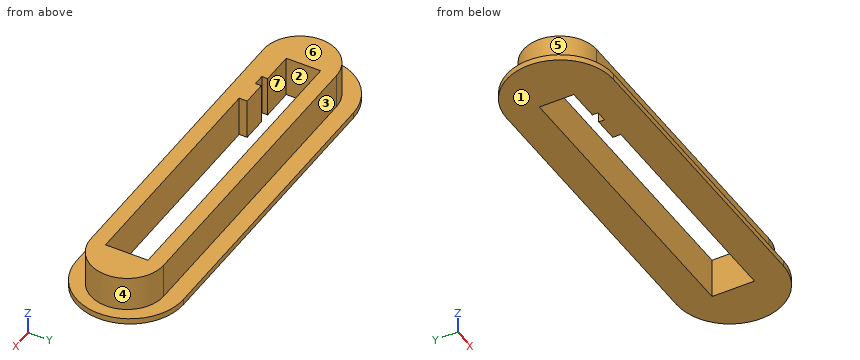
```python
from build123d import *

# Parameters (mm, degrees)
PAD_DEPTH    = 2.1
POCKET_DEPTH = 5
PAD001_DEPTH = 12.5


with BuildPart() as part:
    # Sketch → Pad (new body)
    with BuildSketch(Plane.XY):
        with BuildLine():
            ThreePointArc((0, 19.25), (-19.25, 0), (0, -19.25))
            Line((0, -19.25), (106.5, -19.25))
            ThreePointArc((106.5, -19.25), (125.75, 0), (106.5, 19.25))
            Line((0, 19.25), (106.5, 19.25))
        make_face()
    extrude(amount=PAD_DEPTH)

    # Sketch001 (on Face6 of Pad) → Pocket (cut)
    with BuildSketch(Plane.XY.offset(2.1)):
        Polygon((0.325, 7.65), (108.575, 7.65), (108.575, -7.65), (24.775, -7.65), (24.775, -4.75), (15.975, -4.75), (15.975, -6.85), (11.975, -6.85), (11.975, -4.75), (0.325, -4.75), align=None)
    extrude(amount=-POCKET_DEPTH, mode=Mode.SUBTRACT)

    # Sketch002 (on Face5 of Pocket) → Pad001 (join)
    with BuildSketch(Plane.XY.offset(2.1)):
        with BuildLine():
            ThreePointArc((0, 13.125), (-13.125, 0), (0, -13.125))
            Line((0, -13.125), (108.25, -13.125))
            ThreePointArc((108.25, -13.125), (121.375, 0), (108.25, 13.125))
            Line((0, 13.125), (108.25, 13.125))
        make_face()
        Polygon((0.325, 7.65), (0.325, -4.75), (11.975, -4.75), (11.975, -6.85), (15.975, -6.85), (15.975, -4.75), (24.775, -4.75), (24.775, -7.65), (108.575, -7.65), (108.575, 7.65), align=None, mode=Mode.SUBTRACT)
    extrude(amount=PAD001_DEPTH)


solid = part.part
```
Build history of the part. All positions in model axes, mm. Face numbers are marked on the shaded views. A direction names the side the tool comes from. Round coordinates to 2 decimals unless told otherwise and drop trailing zeros. Loops run counter-clockwise (first coordinate to the right, second up) from the corner with the lowest first, then second, coordinate; pieces in that order, holes last.
Item 1: Two-plate mould, pull along X, no slides. Class the marked faces 4, 5, 6 and 7: released by +X, released by -X, zero draft, split by the parting line, or undercut.
Item 2: Which spindle directions (+Z, -Z, +X, -X, +Y, -Y) get a long thin tool onto all of the face, cutting with end or side? Do the marked faces 1, 2 and 3. Say none if no direction does.
Item 3: Saw through at C-C (z = 7). List the corners of the cut face in (x, y) (3 decimals).
Item 4: Saw through at A-A (y = 0). List the corners of the cut face in (x, z) (3 decimals), then the cut area to 3 significant figures.
Item 5: Saw through at D-D (y = 10). List the corners of the cut face in (x, z), then the cut area to 3 significant figures.
Item 6: Saw through at B-B (x = 104). List the corners of the cut face in (y, z) (3 decimals), then the cut area to 3 significant figures.
Item 7: Pin check, flat tips, straight feed: P1, Ø0.6, axis at y = -6, z = 7, coming from the -X side; P2, Ø8, axis at y = -11.5, z = 1.5, coming from the +X side; P3, Ø6, axis at x = 4.5, z = 9, coming from the +Y side (3 decimals). Stop position of each tip, or through.
Item 8: Drill centre lines: line 1 along Y through (x, z) = (8, 11.25) (3 decimals); line 2 along X through (y, z) = (0.5, 10) (3 decimals); line 3 along Y through (x, z) = (25, 7) (3 decimals). Where is each one in solid material? Low to high.
Worked answers:
1. face 4: released by +X
1. face 5: released by -X
1. face 6: zero draft
1. face 7: undercut
2. face 1: -Z, +X, -X, +Y, -Y
2. face 2: +Z, -Z
2. face 3: +Z, +X, -X, +Y
3. outline: (0, -13.125) - (108.25, -13.125) arc R13.125 ccw to (108.25, 13.125) - (0, 13.125) arc R13.125 ccw to start; hole (0.325, -4.75) - (11.975, -4.75) - (11.975, -6.85) - (15.975, -6.85) - (15.975, -4.75) - (24.775, -4.75) - (24.775, -7.65) - (108.575, -7.65) - (108.575, 7.65) - (0.325, 7.65) - close
4. outline: (-19.25, 0) - (0.325, 0) - (0.325, 14.6) - (-13.125, 14.6) - (-13.125, 2.1) - (-19.25, 2.1) - close; (108.575, 0) - (125.75, 0) - (125.75, 2.1) - (121.375, 2.1) - (121.375, 14.6) - (108.575, 14.6) - close
4. area: 405 mm2
5. outline: (-16.45, 0) - (122.95, 0) - (122.95, 2.1) - (116.75, 2.1) - (116.75, 14.6) - (-8.5, 14.6) - (-8.5, 2.1) - (-16.45, 2.1) - close
5. area: 1,860 mm2
6. outline: (-19.25, 0) - (-7.65, 0) - (-7.65, 14.6) - (-13.125, 14.6) - (-13.125, 2.1) - (-19.25, 2.1) - close; (7.65, 0) - (19.25, 0) - (19.25, 2.1) - (13.125, 2.1) - (13.125, 14.6) - (7.65, 14.6) - close
6. area: 186 mm2
7. P1: stops at x = -11.82
7. P2: stops at x = 124.23
7. P3: stops at y = 13.125
8. line 1: y = -13.125 to -4.75, 7.65 to 13.125
8. line 2: x = -13.115 to 0.325, 108.575 to 121.365
8. line 3: y = -13.125 to -7.65, 7.65 to 13.125
